```python
from build123d import *

# Parameters (mm, degrees)
SKETCH1_W           = 85.8
SKETCH1_H           = 92.5
BOSS_EXTRUDE1_DEPTH = 14.859
SKETCH2_W           = 85.8
SKETCH2_H           = 92.5
SKETCH2_R           = 1
BOSS_EXTRUDE2_DEPTH = 3.175
SKETCH4_W           = 85.8
SKETCH4_H           = 92.5
SKETCH4_W_2         = 75.8
SKETCH4_H_2         = 82.5
BOSS_EXTRUDE3_DEPTH = 5.75
CUT_EXTRUDE1_DEPTH  = 121.870264668
SKETCH5_W           = 14
SKETCH5_H           = 8
CUT_EXTRUDE2_DEPTH  = 121.870264668
SKETCH6_W           = 10
SKETCH6_H           = 6
CUT_EXTRUDE3_DEPTH  = 121.870264668
BOSS_EXTRUDE4_START = 1.9
SKETCH7_R           = 3.54
SKETCH7_R_2         = 1
BOSS_EXTRUDE4_DEPTH = 1.9
FILLET1_R           = 2.5
FILLET2_R           = 2.5
FILLET3_R           = 2.5
FILLET4_R           = 2.5
FILLET5_R           = 2.5
CUT_EXTRUDE4_DEPTH  = 1.5
CUT_EXTRUDE5_DEPTH  = 4
CUT_EXTRUDE7_DEPTH  = 73.9
SKETCH12_W          = 4.501
SKETCH12_H          = 4
BOSS_EXTRUDE8_DEPTH = 5
CUT_EXTRUDE8_DEPTH  = 2.5


with BuildPart() as part:
    # Sketch1 → Boss-Extrude1 (new body)
    with BuildSketch(Plane(origin=(0, 0, 0), x_dir=(1, 0, 0), z_dir=(0, 1, 0))):
        with Locations((37.9, 41.25)):
            Rectangle(SKETCH1_W, SKETCH1_H)
        Polygon((5, 4), (5, 10), (0, 10), (0, 82.5), (70.8, 82.5), (70.8, 79), (75.8, 79), (75.8, 4), (59.9, 4), (59.9, 0), (52.9, 0), (52.9, 4), (41.4, 4), (41.4, 0), (34.4, 0), (34.4, 4), (22.9, 4), (22.9, 0), (15.9, 0), (15.9, 4), align=None, mode=Mode.SUBTRACT)
    extrude(amount=BOSS_EXTRUDE1_DEPTH)

    # Sketch2 → Boss-Extrude2 (add)
    with BuildSketch(Plane(origin=(0, 0, 0), x_dir=(1, 0, 0), z_dir=(0, 1, 0))):
        with Locations((37.9, 41.25)):
            Rectangle(SKETCH2_W, SKETCH2_H)
        with Locations(Location((3.5, 13.5, 0), (0, 0, 270))):
            Circle(SKETCH2_R, mode=Mode.SUBTRACT)
        with Locations(Location((19.4, 3.5, 0), (0, 0, 270))):
            Circle(SKETCH2_R, mode=Mode.SUBTRACT)
        with Locations(Location((37.9, 3.5, 0), (0, 0, 270))):
            Circle(SKETCH2_R, mode=Mode.SUBTRACT)
        with Locations(Location((56.4, 3.5, 0), (0, 0, 270))):
            Circle(SKETCH2_R, mode=Mode.SUBTRACT)
        with Locations(Location((30.3, 56.1, 0), (0, 0, 270))):
            Circle(SKETCH2_R, mode=Mode.SUBTRACT)
        with Locations(Location((71.8, 75.5, 0), (0, 0, 270))):
            Circle(SKETCH2_R, mode=Mode.SUBTRACT)
    extrude(amount=-BOSS_EXTRUDE2_DEPTH)

    # Sketch4 → Boss-Extrude3 (add)
    with BuildSketch(Plane(origin=(0, 14.859, 0), x_dir=(1, 0, 0), z_dir=(0, 1, 0))):
        with Locations((37.9, 41.25)):
            Rectangle(SKETCH4_W, SKETCH4_H)
        with Locations((37.9, 41.25)):
            Rectangle(SKETCH4_W_2, SKETCH4_H_2, mode=Mode.SUBTRACT)
    extrude(amount=BOSS_EXTRUDE3_DEPTH)

    # Sketch3 → Cut-Extrude1 (cut, through all)
    with BuildSketch(Plane(origin=(0, 0, 0), x_dir=(0, 0, -1), z_dir=(1, 0, 0))):
        with BuildLine():
            Line((60.6, 14.859), (60.6, 20.609))
            Line((60.6, 20.609), (51.6, 20.609))
            Line((51.6, 20.609), (51.6, 14.859))
            ThreePointArc((51.6, 14.859), (56.1, 10.359), (60.6, 14.859))
        make_face()
    extrude(amount=-CUT_EXTRUDE1_DEPTH, mode=Mode.SUBTRACT)

    # Sketch5 → Cut-Extrude2 (cut, through all)
    with BuildSketch(Plane.XY):
        with Locations((10.15, 21.25)):
            Rectangle(SKETCH5_W, SKETCH5_H)
        with Locations((28.65, 21.25)):
            Rectangle(SKETCH5_W, SKETCH5_H)
        with Locations((47.15, 21.25)):
            Rectangle(SKETCH5_W, SKETCH5_H)
        with Locations((65.65, 21.25)):
            Rectangle(SKETCH5_W, SKETCH5_H)
    extrude(amount=CUT_EXTRUDE2_DEPTH, mode=Mode.SUBTRACT)

    # Sketch6 → Cut-Extrude3 (cut, through all)
    with BuildSketch(Plane.XY):
        with Locations((59, 20.63)):
            Rectangle(SKETCH6_W, SKETCH6_H)
    extrude(amount=-CUT_EXTRUDE3_DEPTH, mode=Mode.SUBTRACT)

    # Sketch7 → Boss-Extrude4 (add)
    # profile 1 of 6: a face of its own
    with BuildSketch(Plane(origin=(0, 0, 0), x_dir=(1, 0, 0), z_dir=(0, 1, 0)).offset(BOSS_EXTRUDE4_START)):
        with Locations(Location((30.3, 56.1, 0), (0, 0, 90))):
            Circle(SKETCH7_R)
        with Locations(Location((30.3, 56.1, 0), (0, 0, 270))):
            Circle(SKETCH7_R_2, mode=Mode.SUBTRACT)
    # profile 2 of 6: a face of its own
    with BuildSketch(Plane(origin=(0, 0, 0), x_dir=(1, 0, 0), z_dir=(0, 1, 0)).offset(BOSS_EXTRUDE4_START)):
        with BuildLine():
            Line((0, 13.5), (0, 10))
            Line((0, 10), (3.5, 10))
            ThreePointArc((3.5, 10), (5.974873734, 15.974873734), (0, 13.5))
        make_face()
        with Locations(Location((3.5, 13.5, 0), (0, 0, 270))):
            Circle(SKETCH7_R_2, mode=Mode.SUBTRACT)
    # profile 3 of 6: a face of its own
    with BuildSketch(Plane(origin=(0, 0, 0), x_dir=(1, 0, 0), z_dir=(0, 1, 0)).offset(BOSS_EXTRUDE4_START)):
        with BuildLine():
            Line((15.9, 3.5), (15.9, 0))
            Line((15.9, 0), (22.9, 0))
            Line((22.9, 0), (22.9, 3.5))
            ThreePointArc((22.9, 3.5), (19.4, 7), (15.9, 3.5))
        make_face()
        with Locations(Location((19.4, 3.5, 0), (0, 0, 270))):
            Circle(SKETCH7_R_2, mode=Mode.SUBTRACT)
    # profile 4 of 6: a face of its own
    with BuildSketch(Plane(origin=(0, 0, 0), x_dir=(1, 0, 0), z_dir=(0, 1, 0)).offset(BOSS_EXTRUDE4_START)):
        with BuildLine():
            Line((34.4, 3.5), (34.4, 0))
            Line((34.4, 0), (41.4, 0))
            Line((41.4, 0), (41.4, 3.5))
            ThreePointArc((41.4, 3.5), (37.9, 7), (34.4, 3.5))
        make_face()
        with Locations(Location((37.9, 3.5, 0), (0, 0, 270))):
            Circle(SKETCH7_R_2, mode=Mode.SUBTRACT)
    # profile 5 of 6: a face of its own
    with BuildSketch(Plane(origin=(0, 0, 0), x_dir=(1, 0, 0), z_dir=(0, 1, 0)).offset(BOSS_EXTRUDE4_START)):
        with BuildLine():
            Line((52.9, 3.5), (52.9, 0))
            Line((52.9, 0), (59.9, 0))
            Line((59.9, 0), (59.9, 3.5))
            ThreePointArc((59.9, 3.5), (56.4, 7), (52.9, 3.5))
        make_face()
        with Locations(Location((56.4, 3.5, 0), (0, 0, 270))):
            Circle(SKETCH7_R_2, mode=Mode.SUBTRACT)
    # profile 6 of 6: a face of its own
    with BuildSketch(Plane(origin=(0, 0, 0), x_dir=(1, 0, 0), z_dir=(0, 1, 0)).offset(BOSS_EXTRUDE4_START)):
        with BuildLine():
            Line((75.8, 79), (69.863508327, 79))
            ThreePointArc((69.863508327, 79), (69.768493994, 72.054280431), (75.8, 75.5))
            Line((75.8, 75.5), (75.8, 79))
        make_face()
        with Locations(Location((71.8, 75.5, 0), (0, 0, 270))):
            Circle(SKETCH7_R_2, mode=Mode.SUBTRACT)
    extrude(amount=-BOSS_EXTRUDE4_DEPTH)

    # Fillet1
    fillet1_edges = [part.edges().sort_by_distance(p)[0] for p in [
        (-5, 8.717, 5),
    ]]
    fillet(fillet1_edges, radius=FILLET1_R)

    # Fillet2
    fillet2_edges = [part.edges().sort_by_distance(p)[0] for p in [
        (80.8, 8.717, 5),
    ]]
    fillet(fillet2_edges, radius=FILLET2_R)

    # Fillet3
    fillet3_edges = [part.edges().sort_by_distance(p)[0] for p in [
        (80.8, 8.717, -87.5),
    ]]
    fillet(fillet3_edges, radius=FILLET3_R)

    # Fillet4
    fillet4_edges = [part.edges().sort_by_distance(p)[0] for p in [
        (-5, 8.717, -87.5),
    ]]
    fillet(fillet4_edges, radius=FILLET4_R)

    # Fillet5
    fillet5_edges = [part.edges().sort_by_distance(p)[0] for p in [
        (37.9, -3.175, 5),
        (-4.267766953, -3.175, 4.267766953),
        (80.8, -3.175, -41.25),
        (80.067766953, -3.175, 4.267766953),
        (37.9, -3.175, -87.5),
        (80.067766953, -3.175, -86.767766953),
        (-5, -3.175, -41.25),
        (-4.267766953, -3.175, -86.767766953),
    ]]
    fillet(fillet5_edges, radius=FILLET5_R)

    # Sketch8 → Cut-Extrude4 (cut)
    with BuildSketch(Plane(origin=(0, 0, 0), x_dir=(0, 0, -1), z_dir=(1, 0, 0))):
        with BuildLine():
            Line((62.45, 14.855), (62.45, 21.205))
            Line((62.45, 21.205), (49.75, 21.205))
            Line((49.75, 21.205), (49.75, 14.855))
            ThreePointArc((49.75, 14.855), (56.1, 8.505), (62.45, 14.855))
        make_face()
    extrude(amount=-CUT_EXTRUDE4_DEPTH, mode=Mode.SUBTRACT)

    # Sketch9 → Cut-Extrude5 (cut)
    with BuildSketch(Plane(origin=(0, 20.609, 0), x_dir=(1, 0, 0), z_dir=(0, 1, 0))):
        Polygon((3.15, -1.75), (3.15, -3.75), (1.4, -2.75), align=None)
        Polygon((17.15, -1.75), (17.15, -3.75), (18.9, -2.75), align=None)
        Polygon((21.65, -1.75), (21.65, -3.75), (19.9, -2.75), align=None)
        Polygon((35.65, -1.75), (37.4, -2.75), (35.65, -3.75), align=None)
        Polygon((40.15, -1.75), (38.4, -2.75), (40.15, -3.75), align=None)
        Polygon((54.15, -1.75), (54.15, -3.75), (55.9, -2.75), align=None)
        Polygon((58.65, -1.75), (58.65, -3.75), (56.9, -2.75), align=None)
        Polygon((72.65, -1.75), (72.65, -3.75), (74.4, -2.75), align=None)
    extrude(amount=-CUT_EXTRUDE5_DEPTH, mode=Mode.SUBTRACT)

    # Sketch10 → Cut-Extrude7 (cut)
    with BuildSketch(Plane(origin=(0, 0, 0), x_dir=(0, 0, -1), z_dir=(1, 0, 0))):
        Polygon((-3.75, 17.25), (-1.75, 17.25), (-2.75, 15.5), align=None)
    extrude(amount=CUT_EXTRUDE7_DEPTH, mode=Mode.SUBTRACT)

    # Sketch12 → Boss-Extrude8 (add)
    with BuildSketch(Plane.XY):
        with Locations((0.8995, 15.25)):
            Rectangle(SKETCH12_W, SKETCH12_H)
        with Locations((19.3995, 15.25)):
            Rectangle(SKETCH12_W, SKETCH12_H)
        with Locations((37.8995, 15.25)):
            Rectangle(SKETCH12_W, SKETCH12_H)
        with Locations((56.3995, 15.25)):
            Rectangle(SKETCH12_W, SKETCH12_H)
        with Locations((74.9005, 15.25)):
            Rectangle(SKETCH12_W, SKETCH12_H)
    extrude(amount=BOSS_EXTRUDE8_DEPTH)

    # Sketch13 → Cut-Extrude8 (cut)
    with BuildSketch(Plane(origin=(0, 14.859, 0), x_dir=(1, 0, 0), z_dir=(0, 1, 0))):
        with BuildLine():
            Line((3.5, 8.25), (5, 8.25))
            Line((5, 8.25), (5, 5.75))
            Line((5, 5.75), (3.5, 5.75))
            ThreePointArc((3.5, 5.75), (2.25, 7), (3.5, 8.25))
        make_face()
    extrude(amount=-CUT_EXTRUDE8_DEPTH, mode=Mode.SUBTRACT)


solid = part.part
```
Could you check a few things on this model? Use its own coordinates, in mm. A direction names the side the tool comes from. Round coordinates to 2 decimals unless told otherwise and drop trailing zeros. Order: outer loops, then holes, each group sorted by start corner. A loop starts at its lowest first (then second) coordinate and runs counter-clockwise, first axis right, second up. Notation, with made-up numbers: M 34,-32 L 43,-32 A33 cw 43,3 Z; hole C 76.25,28.25 d5. An arc over 180 degrees is marked long. One line per question, with ' | ' between items. Start each with the question number.
(1) For P1, Ø5.5, axis at x = 59, z = -86, coming from the +Y side; P2, Ø7.5, axis at x = 57, z = -4.5, coming from the +Y side; P3, Ø1.5, axis at x = 72, z = -14, coming from the +Y side, each with a flat end and sliding along its axis, tell me the tip position at first contact or that it passes through.
(2) For faces 1 (the face through (39, 1.9, -3)), 2 (the face through (54, 19, -85)), 3 (the face through (-3, 18, -51.6)), which set-ups out of +Z, -Z, +X, -X, +Y, -Y let a thin tool reach every point of the face, with its end or its side?
(3) Suppose I cut it at C-C on x = 66. List the corners of the cut face in (y, z) for me (3 decimals), then the cut area to 3 significant figures.
(4) Suppose I cut it at A-A on y = 3. List the corners of the cut face in (x, z) for me, then the cut area to 3 significant figures.
(5) Please list where these lines run through material, in increasing order: line 1 along X through (y, z) = (0.55, -56.1); line 2 along X through (y, z) = (-1.7, -3.5); line 3 along Z through (x, y) = (20, 5.25).
(6) Thinking about a two-plate mould opening in Z: for faces 4 (the face through (71.8, -0.6, -76.5)), 5 (the face through (38.47, -2.46, 4.25)), 6 (the face through (37, -3.175, -42)), 7 (the face through (56.5, 1, -7)), which applies, +Z half, -Z half, draft (parallel to the pull), parting line (faces both ways), or undercut?
(7) Suppose I cut it at B-B on z = -43.5. List the corners of the cut face in (x, y) for me (3 decimals), then the cut area to 3 significant figures.
Geometry results:
1) P1: y = 17.63 | P2: y = 14.86 | P3: y = 0
2) face 1: +Y | face 2: +Z, -Z, +Y | face 3: -X, +Y
3) outline: M -3.175,-85 A2.5 ccw -0.675,-87.5 L 20.609,-87.5 L 20.609,-82.5 L 0,-82.5 L 0,-4 L 14.859,-4 L 14.859,0 L 17.25,0 L 17.25,1.75 L 15.5,2.75 L 17.25,3.75 L 17.25,5 L -0.675,5 A2.5 ccw -3.175,2.5 Z | area: 538 mm²
4) outline: M -5,-85 A2.5 ccw -2.5,-87.5 L 78.3,-87.5 A2.5 ccw 80.8,-85 L 80.8,2.5 A2.5 ccw 78.3,5 L -2.5,5 A2.5 ccw -5,2.5 Z; hole M 0,-82.5 L 70.8,-82.5 L 70.8,-79 L 75.8,-79 L 75.8,-4 L 59.9,-4 L 59.9,0 L 52.9,0 L 52.9,-4 L 41.4,-4 L 41.4,0 L 34.4,0 L 34.4,-4 L 22.9,-4 L 22.9,0 L 15.9,0 L 15.9,-4 L 5,-4 L 5,-10 L 0,-10 Z | area: 1,940 mm²
5) line 1: -5 to 0, 26.76 to 29.3, 31.3 to 33.84, 75.8 to 80.8 | line 2: -4.78 to 18.4, 20.4 to 36.9, 38.9 to 55.4, 57.4 to 80.58 | line 3: -87.5 to -82.5, 0 to 5
6) face 4: undercut | face 5: +Z half | face 6: draft | face 7: undercut
7) outline: M -5,-0.675 A2.5 ccw -2.5,-3.175 L 78.3,-3.175 A2.5 ccw 80.8,-0.675 L 80.8,20.609 L 75.8,20.609 L 75.8,0 L 0,0 L 0,20.609 L -5,20.609 Z | area: 476 mm²
